The listing builds one solid part. Answer for the finished solid, in the listing's coordinates (mm). Round coordinates to 2 decimals unless told otherwise and drop trailing zeros. Loops run counter-clockwise (first coordinate to the right, second up) from the corner with the lowest first, then second, coordinate; pieces in that order, holes last. Notation, with made-up numbers: (-2.5, -26) -> (46.5, -26) arc R22 ccw to (46.5, -8) -> close; hole circle Ø1 at (-13.75, 80). An arc over 180 degrees is marked (long way). Use a Markdown table: item, result. Add a question column.
Q1. Given pin 1 Ø8 at (x, z) = (365, 4.5) entering from -Y; pin 2 Ø8 at (x, z) = (466, 9.5) entering from -Y; pin 3 Ø1 at (x, z) = (479.5, 13.5) entering from +Y, each flat-ended and moving along its own axis, determine where each tip first touches the part or whether it passes through.
Q2. Consider line 1 (Y direction, x = 288.5, z = 14.5); line 2 (X direction, y = -883, z = 15.5); line 3 (Y direction, x = 22, z = 13.5). Determine where each line is inside the solid, lowest interval first.
Q3. Section A-A on z = 13.5 is taken. Give the vertices of the cut face in (x, y), then the cut area to 3 significant figures.
from build123d import *

# Parameters (mm, degrees)
BOSS_EXTRUDE1_DEPTH = 20
SKETCH3_R           = 10
BOSS_EXTRUDE2_DEPTH = 1240


with BuildPart() as part:
    # Sketch1 → Boss-Extrude1 (new body)
    with BuildSketch(Plane.XY):
        Polygon((0, 0), (-16.689267036, 11.021268793), (-19.444584234, 6.848952034), (-11.099950716, 1.338317638), (-2.755317198, -4.172316759), align=None)
    extrude(amount=BOSS_EXTRUDE1_DEPTH)

    # Sketch3 → Boss-Extrude2 (add)
    with BuildSketch(Plane(origin=(0, 0, 0), x_dir=(-0.866025404, -0.5, 0), z_dir=(0.5, -0.866025404, 0))):
        with Locations((0, -10)):
            Circle(SKETCH3_R)
    extrude(amount=BOSS_EXTRUDE2_DEPTH)


solid = part.part
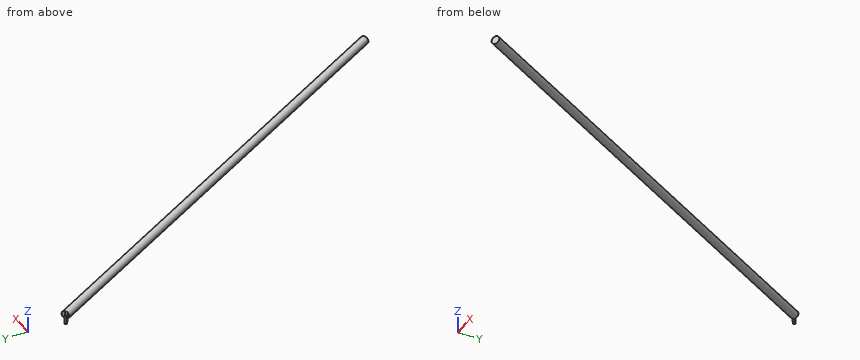
Checked values:
| question | item | result |
|---|---|---|
| 1 | pin 1 | stops at y = -656.97 |
| 1 | pin 2 | stops at y = -834.05 |
| 1 | pin 3 | stops at y = -810.84 |
| 2 | line 1 | y = -517.56 to -481.84 |
| 2 | line 2 | x = 500.16 to 519.44 |
| 2 | line 3 | y = -56.84 to -19.37 |
| 3 | outline | (-19.44, 6.85) -> (-4.84, -2.79) -> (-8.11, -4.68) -> (611.89, -1078.56) -> (628.11, -1069.19) -> (8.11, 4.68) -> (0, 0) -> (-16.69, 11.02) -> close |
| 3 | area | 23,300 mm2 |
